from build123d import *

# Parameters (mm, degrees)
EXTRUDE_1_DEPTH      = 0.6
EXTRUDE_1_DEPTH_BACK = 0.6
SKETCH_1_R           = 1


with BuildPart() as part:
    # 草圖1 → 填料-伸長1 (new, two sides: drawn at the far end of the back side and taken through both)
    with BuildSketch(Plane(origin=(0, 0, 0), x_dir=(0, 0, -1), z_dir=(1, 0, 0)).offset(-EXTRUDE_1_DEPTH_BACK)):
        with BuildLine():
            Line((-4, -10.8801497), (-4, -12.65))
            ThreePointArc((-4, -12.65), (-3.853553391, -13.003553391), (-3.5, -13.15))
            Line((-3.5, -13.15), (-0.185, -13.15))
            Line((-0.185, -13.15), (-0.185, -9.248149815))
            ThreePointArc((-0.185, -9.248149815), (0, 9.25), (0.185, -9.248149815))
            Line((0.185, -9.248149815), (0.185, -13.15))
            Line((0.185, -13.15), (3.5, -13.15))
            ThreePointArc((3.5, -13.15), (3.853553391, -13.003553391), (4, -12.65))
            Line((4, -12.65), (4, -10.8801497))
            ThreePointArc((4, -10.8801497), (4.293177827, -9.837672808), (5.08675807, -9.100827026))
            ThreePointArc((5.08675807, -9.100827026), (5.9e-08, 11.95), (-5.086758175, -9.100826972))
            ThreePointArc((-5.086758175, -9.100826972), (-4.293177858, -9.837672758), (-4, -10.8801497))
        make_face()
        with Locations((2, -11.2)):
            Circle(SKETCH_1_R, mode=Mode.SUBTRACT)
        with Locations((-2, -11.2)):
            Circle(SKETCH_1_R, mode=Mode.SUBTRACT)
    extrude(amount=EXTRUDE_1_DEPTH + EXTRUDE_1_DEPTH_BACK)


solid = part.part
Part model, mm, in its own coordinate system. A direction names the side the tool comes from. Give positions to 0.01 mm unless a question says otherwise; leave off trailing zeros. Order: outer loops, then holes, each group sorted by start corner. A loop starts at its lowest first (then second) coordinate and runs counter-clockwise, first axis right, second up. Notation, with made-up numbers: (47.5, 75) - (85.5, 75) arc R15 ccw to (85.5, 104) - close; hole circle Ø1 at (27, 76). An arc over 180 degrees is marked (long way). One line per question, with ' | ' between items.
1. Band-saw the part on A-A on x = -0.4. List the corners of the cut face in (y, z) (3 decimals), then the cut area to 3 significant figures.
Filled in:
outline: (-13.15, -3.5) arc R0.5 ccw to (-12.65, -4) - (-10.88, -4) arc R2 cw to (-9.101, -5.087) arc R11.14 ccw (long way) to (-9.101, 5.087) arc R2 cw to (-10.88, 4) - (-12.65, 4) arc R0.5 ccw to (-13.15, 3.5) - (-13.15, 0.185) - (-9.248, 0.185) arc R9.25 cw (long way) to (-9.248, -0.185) - (-13.15, -0.185) - close; hole circle Ø2 at (-11.2, -2); hole circle Ø2 at (-11.2, 2) | area: 138 mm²
2. Band-saw the part on C-C on y = -11.2. List the corners of the cut face in (x, z) (3 decimals).
Filled in:
outline: (-0.6, -4) - (0.6, -4) - (0.6, -3) - (-0.6, -3) - close; (-0.6, -1) - (0.6, -1) - (0.6, -0.185) - (-0.6, -0.185) - close; (-0.6, 0.185) - (0.6, 0.185) - (0.6, 1) - (-0.6, 1) - close; (-0.6, 3) - (0.6, 3) - (0.6, 4) - (-0.6, 4) - close
3. Which spindle directions (+Z, -Z, +X, -X, +Y, -Y) get a long thin tool onto all of the face, cutting with end or side? Do faces 4 (the face through (0, -12, -4)), 5 (the face through (0, -11, -0.185)), 6 (the face through (-0.008, -12.176, 2.217)). Say none if no direction does.
Filled in:
face 4: -Z, +X, -X, -Y | face 5: +X, -X, -Y | face 6: +X, -X
4. Band-saw the part on D-D on z = 6.5. List the corners of the cut face in (x, y).
Filled in:
outline: (-0.6, -8.24) - (0.6, -8.24) - (0.6, -6.58) - (-0.6, -6.58) - close; (-0.6, 6.58) - (0.6, 6.58) - (0.6, 9.86) - (-0.6, 9.86) - close
5. Drill centre lines: probe 1 along Y at (x, z) = (-0.1, 2); probe 2 along Y at (x, z) = (0.45, 2.75); probe 3 along Z at (x, y) = (0.2, -8). Where is each one in solid material? Low to high.
Filled in:
probe 1: -13.15 to -12.2, -10.2 to -9.03, 9.03 to 11.77 | probe 2: -13.15 to -11.86, -10.54 to -8.83, 8.83 to 11.61 | probe 3: -6.82 to -4.64, 4.64 to 6.82
6. Drop flat-ended pins along their axis: P1, Ø3, axis at y = -8, z = -3.5, coming from the -X side; P2, Ø0.6, axis at x = 0, y = -12, coming from the +Z side. Give the stop position or say it passes through.
Filled in:
P1: x = -0.6 | P2: z = 4
7. Band-saw the part on B-B on y = -3.5. List the corners of the cut face in (x, z).
Filled in:
outline: (-0.6, -10.27) - (0.6, -10.27) - (0.6, -8.56) - (-0.6, -8.56) - close; (-0.6, 8.56) - (0.6, 8.56) - (0.6, 10.27) - (-0.6, 10.27) - close
8. Pull direction Y, two halves, no side cores. Call faces 1 (the face through (-0.008, -12.176, -1.783)), 2 (the face through (0, -13.15, -2)), 3 (the face through (0, -12, 4)): +Y half, -Y half, draft (parallel to the pull), parting line (faces both ways), or undercut.
Filled in:
face 1: undercut | face 2: -Y half | face 3: draft
